from build123d import *

# Parameters (mm, degrees)
F0_W     = 100
F0_H     = 50
F1_DEPTH = 50
F2_R     = 15
F3_DEPTH = 50
F4_DEPTH = 50


with BuildPart() as f1:
    # F0 (on Top) → F1 (new body)
    with BuildSketch(Plane.XY):
        Rectangle(F0_W, F0_H)
    extrude(amount=F1_DEPTH)

    # F2 (on face) → F3 (cut)
    with BuildSketch(Plane.XY.offset(50)):
        Circle(F2_R)
    extrude(amount=F3_DEPTH, mode=Mode.SUBTRACT)

    # F2 (on face) → F4 (cut)
    with BuildSketch(Plane.XY.offset(50)):
        Circle(F2_R)
    extrude(amount=-F4_DEPTH, mode=Mode.SUBTRACT)


solid = f1.part
Could you check a few things on this model? Use its own coordinates, in mm. Round coordinates to 2 decimals unless told otherwise and drop trailing zeros. Order: outer loops, then holes, each group sorted by start corner. A loop starts at its lowest first (then second) coordinate and runs counter-clockwise, first axis right, second up.
(1) Please list where these lines run through material, in increasing order: line 1 along Y through (x, z) = (0, 29); line 2 along X through (y, z) = (-7, 18); line 3 along X through (y, z) = (1, 46.5).
Response values:
line 1: y = -25 to -15, 15 to 25
line 2: x = -50 to -13.27, 13.27 to 50
line 3: x = -50 to -14.97, 14.97 to 50
(2) Imagine slicing it at A-A (x = 0). Write out the boundary of the cut face in (y, z), plus the area to 3 significant figures.
Response values:
outline: (-25, 0) - (-15, 0) - (-15, 50) - (-25, 50) - close; (15, 0) - (25, 0) - (25, 50) - (15, 50) - close
area: 1,000 mm2
(3) Imagine slicing it at C-C (z = 46.5). Write out the boundary of the cut face in (x, y), plus the area to 3 significant figures.
Response values:
outline: (-50, -25) - (50, -25) - (50, 25) - (-50, 25) - close; hole circle Ø30 at (0, 0)
area: 4,290 mm2
(4) Imagine slicing it at B-B (y = 0). Write out the boundary of the cut face in (x, z).
Response values:
outline: (-50, 0) - (-15, 0) - (-15, 50) - (-50, 50) - close; (15, 0) - (50, 0) - (50, 50) - (15, 50) - close
